Check sheet for the drawn part. Datum: minimum x, y, z corner. Units: mm. A direction names the side the tool comes from. Give positions to 0.01 mm unless a question says otherwise; leave off trailing zeros. Loops run counter-clockwise (first coordinate to the right, second up) from the corner with the lowest first, then second, coordinate; pieces in that order, holes last.
1. Tool access check on the marked faces 1, 2 and 3. Record the directions out of +Z, -Z, +X, -X, +Y, -Y that give a thin tool (end or side, any length) a straight path to the whole face; none if there is none.
2. Material ranges on L1, parallel to X at y = 3, z = 4.25 (1 decimal); L2, parallel to X at y = 2, z = 0.5 (1 decimal); L3, parallel to Z at x = 1.75, y = 2, recorded low to high.
3. Cross-section at D-D, the plane z = 3. Record the cut outline in (x, y), plus the area to 3 significant figures.
4. Cross-section at A-A, the plane y = 10. State how many separate pieces and enclosed holes the cut face has.
5. Go/stop test with flat-tipped pins: pin 1 Ø3 at (x, y) = (3.5, 4) entering from +Z; pin 2 Ø1.5 at (x, y) = (3.13, 2.5) entering from +Z. Record where each tip stops, or that it passes through.
6. Cross-section at C-C, the plane x = 2.75. Record the cut outline in (y, z).
7. Cross-section at B-B, the plane z = 1.25. Record the cut outline in (x, y), plus the area to 3 significant figures.
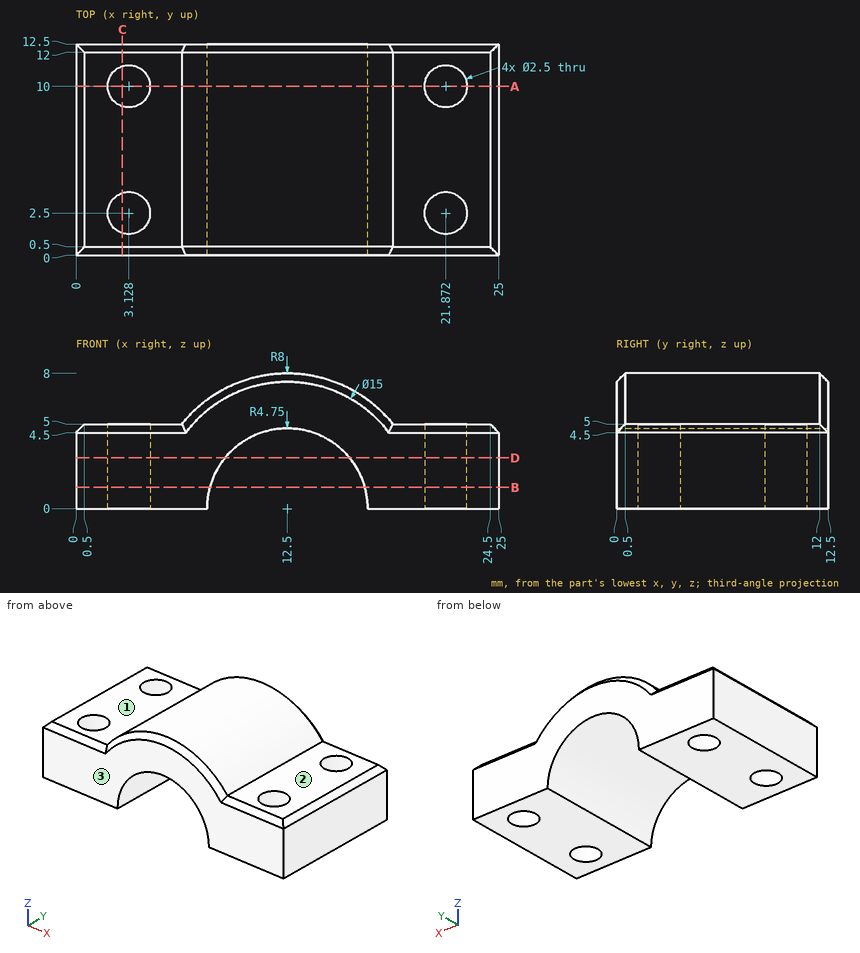
Result:
1. face 1: +Z, -X, +Y, -Y
1. face 2: +Z, +X, +Y, -Y
1. face 3: +Z, -Z, +X, -X, -Y
2. L1: x = 0 to 2, 4.3 to 10.4, 14.6 to 20.7, 23 to 25
2. L2: x = 0 to 2, 4.3 to 7.8, 17.2 to 20.7, 23 to 25
2. L3: z = 0 to 5
3. outline: (0, 0) - (8.82, 0) - (8.82, 12.5) - (0, 12.5) - close; (16.18, 0) - (25, 0) - (25, 12.5) - (16.18, 12.5) - close; hole circle Ø2.5 at (3.13, 2.5); hole circle Ø2.5 at (3.13, 10); hole circle Ø2.5 at (21.87, 2.5); hole circle Ø2.5 at (21.87, 10)
3. area: 201 mm2
4. separate pieces: 3
4. enclosed holes: 0
5. pin 1: stops at z = 5
5. pin 2: passes through
6. outline: (0, 0) - (1.31, 0) - (1.31, 5) - (0.5, 5) - (0, 4.5) - close; (3.69, 0) - (8.81, 0) - (8.81, 5) - (3.69, 5) - close; (11.19, 0) - (12.5, 0) - (12.5, 4.5) - (12, 5) - (11.19, 5) - close
7. outline: (0, 0) - (7.92, 0) - (7.92, 12.5) - (0, 12.5) - close; (17.08, 0) - (25, 0) - (25, 12.5) - (17.08, 12.5) - close; hole circle Ø2.5 at (3.13, 2.5); hole circle Ø2.5 at (3.13, 10); hole circle Ø2.5 at (21.87, 2.5); hole circle Ø2.5 at (21.87, 10)
7. area: 178 mm2
